Build history of the part. All positions in model axes, mm. Give positions to 0.01 mm unless a question says otherwise; leave off trailing zeros. Order: outer loops, then holes, each group sorted by start corner. A loop starts at its lowest first (then second) coordinate and runs counter-clockwise, first axis right, second up. Notation, with made-up numbers: M 18.5,85 L 73.5,85 A28 cw 73.5,105 Z; hole C 51.5,15.5 d11. An arc over 180 degrees is marked long. One line per item, written item: value.
from build123d import *

# Parameters (mm, degrees)
MODEL_R             = 1.5
MODEL_R_2           = 1.3
BOSS_EXTRUDE1_DEPTH = 3


with BuildPart() as part:
    # Model → Boss-Extrude1 (new body)
    with BuildSketch(Plane.XY):
        with BuildLine():
            Line((67.038441792, 41.415856749), (104.038441639, 41.418238239))
            Line((104.038441639, 41.418238239), (108.538521807, 41.418527884))
            ThreePointArc((108.538521807, 41.418527884), (112.537988752, 45.418317376), (108.53819926, 49.417784321))
            Line((108.53819926, 49.417784321), (34.799117207, 50.383081783))
            ThreePointArc((34.799117207, 50.383081783), (32.966554958, 50.620533228), (31.23734869, 51.272080055))
            ThreePointArc((31.23734869, 51.272080055), (28.515998073, 51.939320982), (25.788421234, 51.298006533))
            ThreePointArc((25.788421234, 51.298006533), (24.076314539, 50.668969798), (22.266330888, 50.443236041))
            Line((22.266330888, 50.443236041), (-6.550050988, 50.167207177))
            ThreePointArc((-6.550050988, 50.167207177), (-8.973297656, 49.093954733), (-10.445895761, 46.890446157))
            ThreePointArc((-10.445895761, 46.890446157), (-9.613967932, 43.642213171), (-6.602156551, 42.168403941))
            Line((-6.602156551, 42.168403941), (22.208184202, 41.516932419))
            ThreePointArc((22.208184202, 41.516932419), (24.01842496, 41.280561161), (25.718896078, 40.616301461))
            ThreePointArc((25.718896078, 40.616301461), (28.43787871, 39.93957832), (31.167673514, 40.571275311))
            ThreePointArc((31.167673514, 40.571275311), (32.905215524, 41.200228691), (34.740707643, 41.413777918))
            Line((34.740707643, 41.413777918), (46.038441879, 41.414505092))
            Line((46.038441879, 41.414505092), (56.538441836, 41.415180921))
            Line((56.538441836, 41.415180921), (67.038441792, 41.415856749))
        make_face()
        with Locations((28.487510706, 45.939417458)):
            Circle(MODEL_R, mode=Mode.SUBTRACT)
        with Locations((108.485791619, 45.418177884)):
            Circle(MODEL_R, mode=Mode.SUBTRACT)
        with Locations((-6.485524229, 46.174255041)):
            Circle(MODEL_R_2, mode=Mode.SUBTRACT)
    extrude(amount=BOSS_EXTRUDE1_DEPTH)


solid = part.part
1) Saw through at A-A, the plane z = 1.45. Write the cut outline in (x, y), then the cut area to 3 significant figures.
Check values:
outline: M -10.45,46.89 A4 ccw -6.6,42.17 L 22.21,41.52 A7.54 cw 25.72,40.62 A6 ccw 31.17,40.57 A8 cw 34.74,41.41 L 108.54,41.42 A4 ccw 108.54,49.42 L 34.8,50.38 A8 cw 31.24,51.27 A6 ccw 25.79,51.3 A8.02 cw 22.27,50.44 L -6.55,50.17 A4.76 ccw Z; hole C -6.49,46.17 d2.6; hole C 28.49,45.94 d3; hole C 108.49,45.42 d3
area: 1,030 mm^2
2) Saw through at B-B, the plane x = 74. Write the cut outline in (y, z), then the cut area to 3 significant figures.
Check values:
outline: M 41.42,0 L 49.87,0 L 49.87,3 L 41.42,3 Z
area: 25.4 mm^2
3) Pin check, flat tips, straight feed: pin 1 (0.9 mm diameter, centred on x = 62.5, z = 2, fed in from -Y); pin 2 (1.8 mm diameter, centred on x = 28.49, y = 45.94, fed in from -Z). Stop position of each tip, or through.
Check values:
pin 1: y = 41.42
pin 2: through
4) Drill centre lines: probe 1 along X at (y, z) = (47, 0.6); probe 2 along X at (y, z) = (44.75, 2.5); probe 3 along X at (y, z) = (43.5, 2.55). Where is each one in solid material? Low to high. Write a range as from..to.
Check values:
probe 1: -10.41..-7.49, -5.48..27.43, 29.55..112.21
probe 2: -10.25..27.57, 29.4..107.14, 109.83..112.48
probe 3: -9.49..112.05
5) Mould opens along Y. For faces 1 (the face through (109.917, 45.869, 1.479)), 2 (the face through (23.994, 41.287, 1.479)), 3 (the face through (27.38, 46.95, 1.48)), 4 (the face through (32.992, 50.614, 1.479)) say: released by +Y, released by -Y, zero draft, split by the parting line, or undercut.
Check values:
face 1: undercut
face 2: released by -Y
face 3: undercut
face 4: released by +Y
6) Saw through at C-C, the plane x = 16. Write the cut outline in (y, z).
Check values:
outline: M 41.66,0 L 50.38,0 L 50.38,3 L 41.66,3 Z
